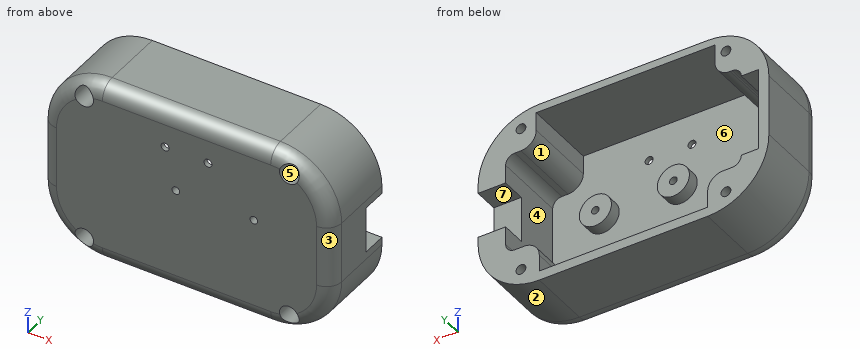
from build123d import *

# Parameters (mm, degrees)
SKETCH2_R           = 1.6
SKETCH2_W           = 24
SKETCH2_H           = 11
SKETCH2_H_2         = 3
SKETCH2_R_2         = 1.25
BOSS_EXTRUDE1_DEPTH = 1.5
BOSS_EXTRUDE2_START = 1.5
SKETCH2_3_R         = 1.6
BOSS_EXTRUDE2_DEPTH = 24
SKETCH3_R           = 5.25
SKETCH3_R_2         = 1.25
BOSS_EXTRUDE3_DEPTH = 4
FILLET1_R           = 10
SKETCH4_R           = 1.3
CUT_EXTRUDE1_DEPTH  = 7
SKETCH5_R           = 3.1
CUT_EXTRUDE2_DEPTH  = 15
FILLET2_R           = 5
SKETCH6_W           = 15
SKETCH6_H           = 9
CUT_EXTRUDE3_DEPTH  = 15
SKETCH7_W           = 12
SKETCH7_H           = 6
CUT_EXTRUDE4_DEPTH  = 15
SKETCH10_W          = 5.662079196
SKETCH10_H          = 27
SKETCH10_W_2        = 55
SKETCH10_H_2        = 10.417373492
CUT_EXTRUDE5_DEPTH  = 24
FILLET6_R           = 5


with BuildPart() as part:
    # Sketch2 → Boss-Extrude1 (new body)
    # profile 1 of 4: a face of its own
    with BuildSketch(Plane(origin=(0, 0, 0), x_dir=(1, 0, 0), z_dir=(0, 1, 0))):
        with BuildLine():
            Line((27.5, 30), (-27.5, 30))
            ThreePointArc((-27.5, 30), (-41.642135624, 24.142135624), (-47.5, 10))
            Line((-47.5, 10), (-47.5, -10))
            ThreePointArc((-47.5, -10), (-41.642135624, -24.142135624), (-27.5, -30))
            Line((-27.5, -30), (27.5, -30))
            ThreePointArc((27.5, -30), (41.642135624, -24.142135624), (47.5, -10))
            Line((47.5, -10), (47.5, 10))
            ThreePointArc((47.5, 10), (41.642135624, 24.142135624), (27.5, 30))
        make_face()
        with Locations(Location((-33.480589606, -24, 0), (0, 0, 270))):
            Circle(SKETCH2_R, mode=Mode.SUBTRACT)
        with Locations(Location((33.480589606, -24, 0), (0, 0, 270))):
            Circle(SKETCH2_R, mode=Mode.SUBTRACT)
        with BuildLine():
            ThreePointArc((-38.5, 13.5), (-37.621320344, 15.621320344), (-35.5, 16.5))
            Line((-35.5, 16.5), (35.5, 16.5))
            ThreePointArc((35.5, 16.5), (37.621320344, 15.621320344), (38.5, 13.5))
            Line((38.5, 13.5), (38.5, -13.5))
            ThreePointArc((38.5, -13.5), (37.621320344, -15.621320344), (35.5, -16.5))
            Line((35.5, -16.5), (12, -16.5))
            Line((12, -16.5), (12, -27.5))
            Line((12, -27.5), (-12, -27.5))
            Line((-12, -27.5), (-12, -16.5))
            Line((-12, -16.5), (-35.5, -16.5))
            ThreePointArc((-35.5, -16.5), (-37.621320344, -15.621320344), (-38.5, -13.5))
            Line((-38.5, -13.5), (-38.5, 13.5))
        make_face(mode=Mode.SUBTRACT)
        with Locations(Location((-33.480589606, 24, 0), (0, 0, 270))):
            Circle(SKETCH2_R, mode=Mode.SUBTRACT)
        with Locations(Location((33.480589606, 24, 0), (0, 0, 270))):
            Circle(SKETCH2_R, mode=Mode.SUBTRACT)
    # profile 2 of 4: a face of its own
    with BuildSketch(Plane(origin=(0, 0, 0), x_dir=(1, 0, 0), z_dir=(0, 1, 0))):
        with Locations((0, -22)):
            Rectangle(SKETCH2_W, SKETCH2_H)
    # profile 3 of 4: a face of its own
    with BuildSketch(Plane(origin=(0, 0, 0), x_dir=(1, 0, 0), z_dir=(0, 1, 0))):
        with Locations((0, -15)):
            Rectangle(SKETCH2_W, SKETCH2_H_2)
    # profile 4 of 4: a face of its own
    with BuildSketch(Plane(origin=(0, 0, 0), x_dir=(1, 0, 0), z_dir=(0, 1, 0))):
        with BuildLine():
            Line((35.5, 16.5), (-35.5, 16.5))
            ThreePointArc((-35.5, 16.5), (-37.621320344, 15.621320344), (-38.5, 13.5))
            Line((-38.5, 13.5), (-38.5, -13.5))
            ThreePointArc((-38.5, -13.5), (-37.621320344, -15.621320344), (-35.5, -16.5))
            Line((-35.5, -16.5), (-12, -16.5))
            Line((-12, -16.5), (-12, -13.5))
            Line((-12, -13.5), (12, -13.5))
            Line((12, -13.5), (12, -16.5))
            Line((12, -16.5), (35.5, -16.5))
            ThreePointArc((35.5, -16.5), (37.621320344, -15.621320344), (38.5, -13.5))
            Line((38.5, -13.5), (38.5, 13.5))
            ThreePointArc((38.5, 13.5), (37.621320344, 15.621320344), (35.5, 16.5))
        make_face()
        with Locations(Location((-3.480589606, -4, 0), (0, 0, 270))):
            Circle(SKETCH2_R_2, mode=Mode.SUBTRACT)
        with Locations(Location((22, -4, 0), (0, 0, 270))):
            Circle(SKETCH2_R_2, mode=Mode.SUBTRACT)
    extrude(amount=BOSS_EXTRUDE1_DEPTH)

    # Sketch2<3> → Boss-Extrude2 (add)
    with BuildSketch(Plane(origin=(0, 0, 0), x_dir=(1, 0, 0), z_dir=(0, 1, 0)).offset(BOSS_EXTRUDE2_START)):
        with BuildLine():
            Line((27.5, 30), (-27.5, 30))
            ThreePointArc((-27.5, 30), (-41.642135624, 24.142135624), (-47.5, 10))
            Line((-47.5, 10), (-47.5, -10))
            ThreePointArc((-47.5, -10), (-41.642135624, -24.142135624), (-27.5, -30))
            Line((-27.5, -30), (27.5, -30))
            ThreePointArc((27.5, -30), (41.642135624, -24.142135624), (47.5, -10))
            Line((47.5, -10), (47.5, 10))
            ThreePointArc((47.5, 10), (41.642135624, 24.142135624), (27.5, 30))
        make_face()
        with Locations(Location((-33.480589606, -24, 0), (0, 0, 270))):
            Circle(SKETCH2_3_R, mode=Mode.SUBTRACT)
        with Locations(Location((33.480589606, -24, 0), (0, 0, 270))):
            Circle(SKETCH2_3_R, mode=Mode.SUBTRACT)
        with BuildLine():
            ThreePointArc((-38.5, 13.5), (-37.621320344, 15.621320344), (-35.5, 16.5))
            Line((-35.5, 16.5), (35.5, 16.5))
            ThreePointArc((35.5, 16.5), (37.621320344, 15.621320344), (38.5, 13.5))
            Line((38.5, 13.5), (38.5, -13.5))
            ThreePointArc((38.5, -13.5), (37.621320344, -15.621320344), (35.5, -16.5))
            Line((35.5, -16.5), (12, -16.5))
            Line((12, -16.5), (12, -27.5))
            Line((12, -27.5), (-12, -27.5))
            Line((-12, -27.5), (-12, -16.5))
            Line((-12, -16.5), (-35.5, -16.5))
            ThreePointArc((-35.5, -16.5), (-37.621320344, -15.621320344), (-38.5, -13.5))
            Line((-38.5, -13.5), (-38.5, 13.5))
        make_face(mode=Mode.SUBTRACT)
        with Locations(Location((-33.480589606, 24, 0), (0, 0, 270))):
            Circle(SKETCH2_3_R, mode=Mode.SUBTRACT)
        with Locations(Location((33.480589606, 24, 0), (0, 0, 270))):
            Circle(SKETCH2_3_R, mode=Mode.SUBTRACT)
    extrude(amount=BOSS_EXTRUDE2_DEPTH)

    # Sketch3 → Boss-Extrude3 (add)
    # profile 1 of 2: a face of its own
    with BuildSketch(Plane(origin=(0, 1.5, 0), x_dir=(1, 0, 0), z_dir=(0, 1, 0))):
        with Locations(Location((-3.480589606, -4, 0), (0, 0, 270))):
            Circle(SKETCH3_R)
        with Locations(Location((-3.480589606, -4, 0), (0, 0, 270))):
            Circle(SKETCH3_R_2, mode=Mode.SUBTRACT)
    # profile 2 of 2: a face of its own
    with BuildSketch(Plane(origin=(0, 1.5, 0), x_dir=(1, 0, 0), z_dir=(0, 1, 0))):
        with Locations(Location((22, -4, 0), (0, 0, 270))):
            Circle(SKETCH3_R)
        with Locations(Location((22, -4, 0), (0, 0, 270))):
            Circle(SKETCH3_R_2, mode=Mode.SUBTRACT)
    extrude(amount=BOSS_EXTRUDE3_DEPTH)

    # Fillet1
    fillet1_edges = [part.edges().sort_by_distance(p)[0] for p in [
        (-12, 13.5, 16.5),
        (12, 13.5, 16.5),
    ]]
    fillet(fillet1_edges, radius=FILLET1_R)

    # Sketch4 → Cut-Extrude1 (cut)
    with BuildSketch(Plane(origin=(0, 1.5, 0), x_dir=(1, 0, 0), z_dir=(0, 1, 0))):
        with Locations(Location((-7, -17.5, 0), (0, 0, 270))):
            Circle(SKETCH4_R)
        with Locations(Location((7, -17.5, 0), (0, 0, 270))):
            Circle(SKETCH4_R)
    extrude(amount=-CUT_EXTRUDE1_DEPTH, mode=Mode.SUBTRACT)

    # Sketch5 → Cut-Extrude2 (cut)
    with BuildSketch(Plane.XZ):
        with Locations(Location((-33.480589606, 24, 0), (0, 0, 270))):
            Circle(SKETCH5_R)
        with Locations(Location((-33.480589606, -24, 0), (0, 0, 270))):
            Circle(SKETCH5_R)
        with Locations(Location((33.480589606, -24, 0), (0, 0, 270))):
            Circle(SKETCH5_R)
        with Locations(Location((33.480589606, 24, 0), (0, 0, 270))):
            Circle(SKETCH5_R)
    extrude(amount=-CUT_EXTRUDE2_DEPTH, mode=Mode.SUBTRACT)

    # Fillet2
    # the kernel refuses this fillet: 5 mm, written as the material it takes off along each edge
    with BuildSketch(Plane(origin=(27.5, 0, -10), x_dir=(1, 0, 0), z_dir=(0, 0, 1))) as fillet2_piece_1:
        with BuildLine():
            CenterArc((20 - FILLET2_R, FILLET2_R), FILLET2_R, 270, 90)
            Line((20, FILLET2_R), (20, 0))
            Line((20, 0), (20 - FILLET2_R, 0))
        make_face()
    revolve(axis=Axis((27.5, 0, -10), (0, 1, 0)), revolution_arc=90, mode=Mode.SUBTRACT)
    with BuildSketch(Plane(origin=(47.5, 0, 10), x_dir=(-1, 0, 0), z_dir=(0, 0, -1)), Plane(origin=(-47.5, 0, -10), x_dir=(1, 0, 0), z_dir=(0, 0, 1))) as fillet2_piece_2:
        with BuildLine():
            CenterArc((FILLET2_R, FILLET2_R), FILLET2_R, 180, 90)
            Line((0, FILLET2_R), (0, 0))
            Line((0, 0), (FILLET2_R, 0))
        make_face()
    extrude(amount=20, mode=Mode.SUBTRACT)
    with BuildSketch(Plane(origin=(27.5, 0, 10), x_dir=(0, 0, 1), z_dir=(-1, 0, 0))) as fillet2_piece_3:
        with BuildLine():
            CenterArc((20 - FILLET2_R, FILLET2_R), FILLET2_R, 270, 90)
            Line((20, FILLET2_R), (20, 0))
            Line((20, 0), (20 - FILLET2_R, 0))
        make_face()
    revolve(axis=Axis((27.5, 0, 10), (0, 1, 0)), revolution_arc=90, mode=Mode.SUBTRACT)
    with BuildSketch(Plane(origin=(-27.5, 0, 30), x_dir=(0, 0, -1), z_dir=(1, 0, 0)), Plane(origin=(27.5, 0, -30), x_dir=(0, 0, 1), z_dir=(-1, 0, 0))) as fillet2_piece_4:
        with BuildLine():
            CenterArc((FILLET2_R, FILLET2_R), FILLET2_R, 180, 90)
            Line((0, FILLET2_R), (0, 0))
            Line((0, 0), (FILLET2_R, 0))
        make_face()
    extrude(amount=55, mode=Mode.SUBTRACT)
    with BuildSketch(Plane(origin=(-27.5, 0, 10), x_dir=(-1, 0, 0), z_dir=(0, 0, -1))) as fillet2_piece_5:
        with BuildLine():
            CenterArc((20 - FILLET2_R, FILLET2_R), FILLET2_R, 270, 90)
            Line((20, FILLET2_R), (20, 0))
            Line((20, 0), (20 - FILLET2_R, 0))
        make_face()
    revolve(axis=Axis((-27.5, 0, 10), (0, 1, 0)), revolution_arc=90, mode=Mode.SUBTRACT)
    with BuildSketch(Plane(origin=(-27.5, 0, -10), x_dir=(0, 0, -1), z_dir=(1, 0, 0))) as fillet2_piece_6:
        with BuildLine():
            CenterArc((20 - FILLET2_R, FILLET2_R), FILLET2_R, 270, 90)
            Line((20, FILLET2_R), (20, 0))
            Line((20, 0), (20 - FILLET2_R, 0))
        make_face()
    revolve(axis=Axis((-27.5, 0, -10), (0, 1, 0)), revolution_arc=90, mode=Mode.SUBTRACT)

    # Sketch6 → Cut-Extrude3 (cut)
    with BuildSketch(Plane(origin=(47.5, 0, 0), x_dir=(0, 0, -1), z_dir=(1, 0, 0))):
        with Locations((0, 22)):
            Rectangle(SKETCH6_W, SKETCH6_H)
    extrude(amount=-CUT_EXTRUDE3_DEPTH, mode=Mode.SUBTRACT)

    # Sketch7 → Cut-Extrude4 (cut)
    with BuildSketch(Plane(origin=(0, 25.5, 0), x_dir=(1, 0, 0), z_dir=(0, 1, 0))):
        with Locations((22.5, -19.5)):
            Rectangle(SKETCH7_W, SKETCH7_H)
    extrude(amount=-CUT_EXTRUDE4_DEPTH, mode=Mode.SUBTRACT)

    # Sketch10 → Cut-Extrude5 (cut)
    with BuildSketch(Plane(origin=(0, 25.5, 0), x_dir=(1, 0, 0), z_dir=(0, 1, 0))):
        with Locations((-41.331039598, 0)):
            Rectangle(SKETCH10_W, SKETCH10_H)
        with Locations((0, 21.708686746)):
            Rectangle(SKETCH10_W_2, SKETCH10_H_2)
        with BuildLine():
            Line((-22, -16.5), (-29.856380317, -16.5))
            Line((-29.856380317, -16.5), (-29.856380317, -27.5))
            Line((-29.856380317, -27.5), (-12, -27.5))
            Line((-12, -27.5), (-12, -26.5))
            ThreePointArc((-12, -26.5), (-14.928932188, -19.428932188), (-22, -16.5))
        make_face()
        with BuildLine():
            Line((-12, -16.5), (-22, -16.5))
            ThreePointArc((-22, -16.5), (-14.928932188, -19.428932188), (-12, -26.5))
            Line((-12, -26.5), (-12, -16.5))
        make_face()
        with BuildLine():
            Line((12, -16.5), (12, -26.5))
            ThreePointArc((12, -26.5), (13.196591569, -21.75658351), (16.5, -18.148353456))
            Line((16.5, -18.148353456), (16.5, -22.5))
            Line((16.5, -22.5), (28.5, -22.5))
            Line((28.5, -22.5), (28.5, -16.5))
            Line((28.5, -16.5), (12, -16.5))
        make_face()
        with BuildLine():
            Line((12, -26.5), (12, -27.5))
            Line((12, -27.5), (28.5, -27.5))
            Line((28.5, -27.5), (28.5, -22.5))
            Line((28.5, -22.5), (16.5, -22.5))
            Line((16.5, -22.5), (16.5, -18.148353456))
            ThreePointArc((16.5, -18.148353456), (13.196591569, -21.75658351), (12, -26.5))
        make_face()
    extrude(amount=-CUT_EXTRUDE5_DEPTH, mode=Mode.SUBTRACT)

    # Fillet6
    fillet6_edges = [part.edges().sort_by_distance(p)[0] for p in [
        (28.5, 13.5, 16.5),
        (-29.856380317, 13.5, 16.5),
        (27.5, 13.5, -16.5),
        (-27.5, 13.5, -16.5),
    ]]
    fillet(fillet6_edges, radius=FILLET6_R)


solid = part.part
The model under review builds one solid part; all positions refer to its coordinate system, in mm. Face numbers are marked on the shaded views. A direction names the side the tool comes from. Round coordinates to 2 decimals unless told otherwise and drop trailing zeros. Order: outer loops, then holes, each group sorted by start corner. A loop starts at its lowest first (then second) coordinate and runs counter-clockwise, first axis right, second up. Notation, with made-up numbers: (57.5, 14.25) -> (100.5, 14.25) arc R28 cw to (100.5, 52.25) -> close; hole circle Ø6 at (64, 12.5). An arc over 180 degrees is marked (long way). Use CSV: the item, a comma, the result in double quotes. Start each with the question number.
(1) Insertion check: pin 1 (10 mm diameter, centred on x = -31, z = 9.5, fed in from +Y); pin 2 (2.5 mm diameter, centred on x = 41, y = 22, fed in from -Z); pin 3 (3 mm diameter, centred on x = 22.5, z = -22.5, fed in from -Y); pin 4 (1.7 mm diameter, centred on x = -40.5, y = 16.5, fed in from -Z). Each pin has a flat end and moves straight along its axis. Give the tip position at first contact, or say it passes through.
(2) Tool access review of the marked faces 5, 6 and 7: name each direction out of +Z, -Z, +X, -X, +Y, -Y from which nothing blocks a thin tool from reaching the whole face with its end or side.
(3) Consider section B-B on z = -5. Write out the cut boundary in (x, y).
(4) Mouldability with a two-part tool opening along Z and no side actions: class the marked faces 1, 2, 3 and 4 as pulls with the +Z half, pulls with the -Z half, needs draft (parallel to the pull), parting line crosses it, or undercut.
(5) Wall thickness on probe 1 along Z at (x, y) = (-13.5, 22.5); probe 2 along X at (y, z) = (11.5, 24); probe 3 along X at (y, z) = (17, 24): over which ranges is each line inside the solid? List them lowest first. Write a range as from..to.
(6) Consider section A-A on x = 7. Write out the cut boundary in (y, z).
(7) Consider section C-C on x = -23. Write out the cut boundary in (y, z).
(8) Consider section D-D on y = 10.75. State how many separate pieces and enclosed holes the cut face has, and give its area (3 significant figures).
Responses:
1,pin 1,"y = 1.5"
1,pin 2,"z = -25.81"
1,pin 3,"y = 0"
1,pin 4,"z = -25.89"
2,face 5,"-Y"
2,face 6,"+Y"
2,face 7,"+X, +Y"
3,outline,"(-47.5, 5) arc R5 ccw to (-42.5, 0) -> (42.5, 0) arc R5 ccw to (47.5, 5) -> (47.5, 17.5) -> (38.5, 17.5) -> (38.5, 1.5) -> (-44.16, 1.5) -> (-44.16, 25.5) -> (-47.5, 25.5) -> close"
4,face 1,"undercut"
4,face 2,"pulls with the -Z half"
4,face 3,"needs draft"
4,face 4,"undercut"
5,probe 1,"-30..-26.92, 27.5..30"
5,probe 2,"-41.78..-36.58, -30.38..-29.86, 28.5..30.38, 36.58..41.78"
5,probe 3,"-41.78..-35.08, -31.88..-29.86, 28.5..31.88, 35.08..41.78"
6,outline,"(0, -25) arc R5 ccw to (5, -30) -> (25.5, -30) -> (25.5, -26.92) -> (1.5, -26.92) -> (1.5, 16.2) -> (0, 16.2) -> close; (0, 18.8) -> (1.5, 18.8) -> (1.5, 27.5) -> (25.5, 27.5) -> (25.5, 30) -> (5, 30) arc R5 ccw to (0, 25) -> close"
7,outline,"(0, -25) arc R5 ccw to (5, -30) -> (25.5, -30) -> (25.5, -26.92) -> (1.5, -26.92) -> (1.5, 27.5) -> (25.5, 27.5) -> (25.5, 30) -> (5, 30) arc R5 ccw to (0, 25) -> close"
8,separate pieces,"1"
8,enclosed holes,"5"
8,area,"1,310 mm²"
